Check sheet for the modelled part. Datum: model origin and axes. Units: mm. A direction names the side the tool comes from. Give positions to 0.01 mm unless a question says otherwise; leave off trailing zeros. Write each loop counter-clockwise with the first axis right and the second up, starting at its lowest first coordinate (ties: lowest second). Pieces come first, ordered by that corner, then holes. Notation, with made-up numbers: (16.25, 79) -> (20.25, 79) arc R33 ccw to (20.25, 108) -> close; hole circle Ø8 at (0.25, 13). An arc over 180 degrees is marked (long way). Use a Markdown table: item, result. Add a question column.
1. Scan lines: probe 1 along X at (y, z) = (-31.5, 0.85); probe 2 along Y at (x, z) = (0.5, 1.3). Record each from-to range of solid material in increasing order. Write a range as [from, to].
2. Cross-section at B-B (y = -30). Enter the section's corners in (x, z).
3. Release check for a two-part mould opening along X. For faces 1 (the flat face through (-65, 2, 0)), 2 (the flat face through (10, -30, 0)), 3 (the flat face through (-1, 1, -2.5)), 4 (the flat face through (-10, -30, 0)) record: released by +X, released by -X, zero draft, split by the parting line, or undercut.
4. Cross-section at A-A (x = -8). Enter the section's corners in (y, z).
5. Set-up check for faces 5 (the flat face through (0, -28, 0)), 6 (the flat face through (65, 2, 0)): record each of +Z, -Z, +X, -X, +Y, -Y from which the full face is reachable in a straight line by a thin tool's end or side.
from build123d import *

# Parameters (mm, degrees)
SKETCH2_W           = 130
SKETCH2_H           = 100
BOSS_EXTRUDE1_DEPTH = 2.5
FILLET1_R           = 5
SKETCH3_W           = 20
SKETCH3_H           = 4
CUT_EXTRUDE1_DEPTH  = 5


with BuildPart() as part:
    # Sketch2 → Boss-Extrude1 (new body, symmetric)
    with BuildSketch(Plane.XY):
        Rectangle(SKETCH2_W, SKETCH2_H)
    extrude(amount=BOSS_EXTRUDE1_DEPTH, both=True)

    # Fillet1
    fillet1_edges = [part.edges().sort_by_distance(p)[0] for p in [
        (-65, -50, 0),
        (65, -50, 0),
    ]]
    fillet(fillet1_edges, radius=FILLET1_R)

    # Sketch3 → Cut-Extrude1 (cut)
    with BuildSketch(Plane.XY.offset(2.5)):
        with Locations((0, -30)):
            Rectangle(SKETCH3_W, SKETCH3_H)
    extrude(amount=-CUT_EXTRUDE1_DEPTH, mode=Mode.SUBTRACT)


solid = part.part
Worked answers:
| question | item | result |
|---|---|---|
| 1 | probe 1 | x = [-65, -10], [10, 65] |
| 1 | probe 2 | y = [-50, -32], [-28, 50] |
| 2 | outline | (-65, -2.5) -> (-10, -2.5) -> (-10, 2.5) -> (-65, 2.5) -> close; (10, -2.5) -> (65, -2.5) -> (65, 2.5) -> (10, 2.5) -> close |
| 3 | face 1 | released by -X |
| 3 | face 2 | undercut |
| 3 | face 3 | zero draft |
| 3 | face 4 | undercut |
| 4 | outline | (-50, -2.5) -> (-32, -2.5) -> (-32, 2.5) -> (-50, 2.5) -> close; (-28, -2.5) -> (50, -2.5) -> (50, 2.5) -> (-28, 2.5) -> close |
| 5 | face 5 | +Z, -Z |
| 5 | face 6 | +Z, -Z, +X, +Y, -Y |
